Here's how the part is built. I have some questions about the finished solid (model axes, mm). Face numbers are marked on the shaded views. A direction names the side the tool comes from. Give positions to 0.01 mm unless a question says otherwise; leave off trailing zeros. Loops run counter-clockwise (first coordinate to the right, second up) from the corner with the lowest first, then second, coordinate; pieces in that order, holes last. Notation, with made-up numbers: (-23.75, 8.25) - (28.25, 8.25) arc R19 ccw to (28.25, 31.25) - close; hole circle Ø7 at (84.5, -10.75). An arc over 180 degrees is marked (long way). Use a Markdown table: item, result.
from build123d import *

# Parameters (mm, degrees)
BOSS_EXTRU_1_DEPTH           = 20
ENL_V_MAT_EXTRU_1_DEPTH      = 127.792788454
ENL_V_MAT_EXTRU_1_DEPTH_BACK = 127.792788454
ESQUISSE4_R                  = 2.25
CHANFREIN1_SIZE              = 2


with BuildPart() as part:
    # Esquisse3 → Boss.-Extru.1 (new body)
    with BuildSketch(Plane.XY):
        with BuildLine():
            Line((0, -100.352508149), (0, -29.115804262))
            ThreePointArc((0, -29.115804262), (0.779317725, -25.671715487), (2.965436872, -22.89863657))
            Line((2.965436872, -22.89863657), (28.598971382, -2.141009609))
            ThreePointArc((28.598971382, -2.141009609), (40.22943243, -2.99679919), (38.648412133, -14.551035418))
            Line((38.648412133, -14.551035418), (11.974077654, -36.151485576))
            ThreePointArc((11.974077654, -36.151485576), (10.334488294, -38.231294764), (9.75, -40.814361345))
            Line((9.75, -40.814361345), (9.75, -54.752508149))
            ThreePointArc((9.75, -54.752508149), (10.482858086, -57.605686201), (12.5, -59.752508149))
            ThreePointArc((12.5, -59.752508149), (14.517141914, -61.899330096), (15.25, -64.752508149))
            Line((15.25, -64.752508149), (15.25, -100.252508149))
            ThreePointArc((15.25, -100.252508149), (20.99, -105.992508149), (26.73, -100.252508149))
            Line((26.73, -100.252508149), (26.73, -88.352508149))
            ThreePointArc((26.73, -88.352508149), (33.99, -81.092508149), (41.25, -88.352508149))
            Line((41.25, -88.352508149), (41.25, -100.352508149))
            ThreePointArc((41.25, -100.352508149), (20.625, -120.977508149), (0, -100.352508149))
        make_face()
        with BuildLine():
            Line((4.5, -100.352508149), (4.5, -29.115804262))
            ThreePointArc((4.5, -29.115804262), (4.840951505, -27.609015423), (5.797378631, -26.395793396))
            Line((5.797378631, -26.395793396), (31.562630973, -5.531503439))
            ThreePointArc((31.562630973, -5.531503439), (36.732275603, -5.82874095), (35.948188205, -10.947215595))
            Line((35.948188205, -10.947215595), (9.142135894, -32.654328749))
            ThreePointArc((9.142135894, -32.654328749), (6.272854514, -36.293994828), (5.25, -40.814361345))
            Line((5.25, -40.814361345), (5.25, -54.752508149))
            ThreePointArc((5.25, -54.752508149), (6.539886497, -59.774320575), (10.090211132, -63.552892026))
            ThreePointArc((10.090211132, -63.552892026), (10.574170325, -64.06796447), (10.75, -64.752508149))
            Line((10.75, -64.752508149), (10.75, -100.252508149))
            ThreePointArc((10.75, -100.252508149), (20.99, -110.492508149), (31.23, -100.252508149))
            Line((31.23, -100.252508149), (31.23, -88.352508149))
            ThreePointArc((31.23, -88.352508149), (33.99, -85.592508149), (36.75, -88.352508149))
            Line((36.75, -88.352508149), (36.75, -100.352508149))
            ThreePointArc((36.75, -100.352508149), (20.625, -116.477508149), (4.5, -100.352508149))
        make_face(mode=Mode.SUBTRACT)
    extrude(amount=BOSS_EXTRU_1_DEPTH)

    # Esquisse4 → Enlèv. mat.-Extru.1 (cut, two sides: drawn at the far end of the back side and taken through both)
    with BuildSketch(Plane(origin=(9.75, 0, 0), x_dir=(0, 0, -1), z_dir=(1, 0, 0)).offset(-ENL_V_MAT_EXTRU_1_DEPTH_BACK)):
        with Locations(Location((-10, -47.783434747, 0), (0, 0, 90))):
            Circle(ESQUISSE4_R)
    extrude(amount=ENL_V_MAT_EXTRU_1_DEPTH + ENL_V_MAT_EXTRU_1_DEPTH_BACK, mode=Mode.SUBTRACT)

    # Chanfrein1
    chanfrein1_edges = [part.edges().sort_by_distance(p)[0] for p in [
        (9.75, -50.033434747, 10),
    ]]
    chamfer(chanfrein1_edges, length=CHANFREIN1_SIZE)


solid = part.part
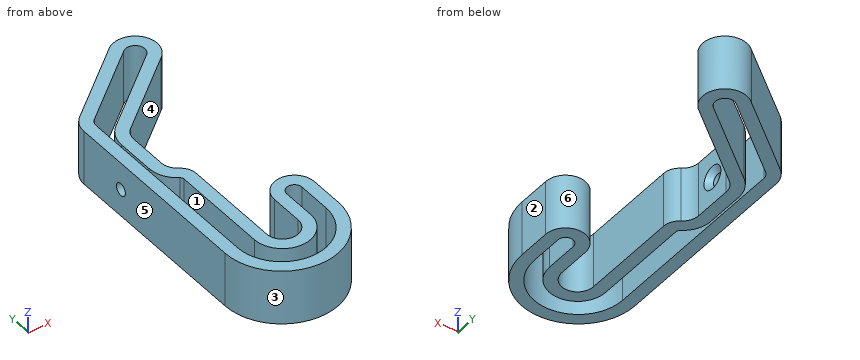
(1) Suppose I cut it at A-A on y = -70.5. Write out the boundary of the cut face in (x, z).
A:
| item | result |
|---|---|
| outline | (0, 0) - (4.5, 0) - (4.5, 20) - (0, 20) - close; (10.75, 0) - (15.25, 0) - (15.25, 20) - (10.75, 20) - close |
(2) On a 3-axis mill with a long thin cutter (end or side, diameter ignored), from which of +Z, -Z, +X, -X, +Y, -Y can I reach the whole of each face in a straight line? I mean the marked faces 1, 2 and 3. Say none if no direction works.
A:
| item | result |
|---|---|
| face 1 | +Z, -Z |
| face 2 | +Z, -Z, +X, -Y |
| face 3 | +Z, -Z, -Y |
(3) Suppose I cut it at B-B on x = 21. Write out the boundary of the cut face in (y, z), plus the area to 3 significant figures.
A:
| item | result |
|---|---|
| outline | (-120.97, 0) - (-116.47, 0) - (-116.47, 20) - (-120.97, 20) - close; (-110.49, 0) - (-105.99, 0) - (-105.99, 20) - (-110.49, 20) - close; (-28.84, 0) - (-23.05, 0) - (-23.05, 20) - (-28.84, 20) - close; (-14.08, 0) - (-8.29, 0) - (-8.29, 20) - (-14.08, 20) - close |
| area | 412 mm2 |
(4) If I drill on line 1 (X direction, y = -91, z = 16); line 2 (X direction, y = -84, z = 14.5); line 3 (Y direction, x = 27.5, z = 18.5), over which ranges is the centre line in solid material (lowest first)?
A:
| item | result |
|---|---|
| line 1 | 0 to 4.5, 10.75 to 15.25, 26.73 to 31.23, 36.75 to 41.25 |
| line 2 | 0 to 4.5, 10.75 to 15.25, 28.18 to 39.8 |
| line 3 | -119.8 to -114.94, -108.16 to -85.1, -23.58 to -17.79, -8.82 to -3.03 |
(5) Suppose I cut it at D-D on y = -7.5. Write out the boundary of the cut face in (x, z), plus the area to 3 significant figures.
A:
| item | result |
|---|---|
| outline | (21.98, 0) - (29.13, 0) - (29.13, 20) - (21.98, 20) - close; (37.47, 0) - (41.99, 0) - (41.99, 20) - (37.47, 20) - close |
| area | 233 mm2 |
(6) We'd pull the mould along X, two halves only. Please class the marked faces 4, 5 and 6: pulls with the +X half, pulls with the -X half, needs draft (parallel to the pull), parting line crosses it, or undercut.
A:
| item | result |
|---|---|
| face 4 | pulls with the +X half |
| face 5 | pulls with the -X half |
| face 6 | undercut |
(7) Suppose I cut it at C-C on y = -103. Write out the boundary of the cut face in (x, z), plus the area to 3 significant figures.
A:
| item | result |
|---|---|
| outline | (0.17, 0) - (4.72, 0) - (4.72, 20) - (0.17, 20) - close; (11.13, 0) - (15.95, 0) - (15.95, 20) - (11.13, 20) - close; (26.03, 0) - (30.85, 0) - (30.85, 20) - (26.03, 20) - close; (36.53, 0) - (41.08, 0) - (41.08, 20) - (36.53, 20) - close |
| area | 375 mm2 |
(8) Will these pins go through, and if not, where does the flat tip stop? pin 1 (10 mm diameter, centred on y = -74, z = 6.5, fed in from +X); pin 2 (10 mm diameter, centred on y = -85.5, z = 17, fed in from +X); pin 3 (2 mm diameter, centred on x = 28, y = -27, fed in from +Z); pin 4 (10 mm diameter, centred on y = -49, z = 10.5, fed in from +X).
A:
| item | result |
|---|---|
| pin 1 | x = 15.25 |
| pin 2 | x = 41.25 |
| pin 3 | through |
| pin 4 | x = 9.75 |
